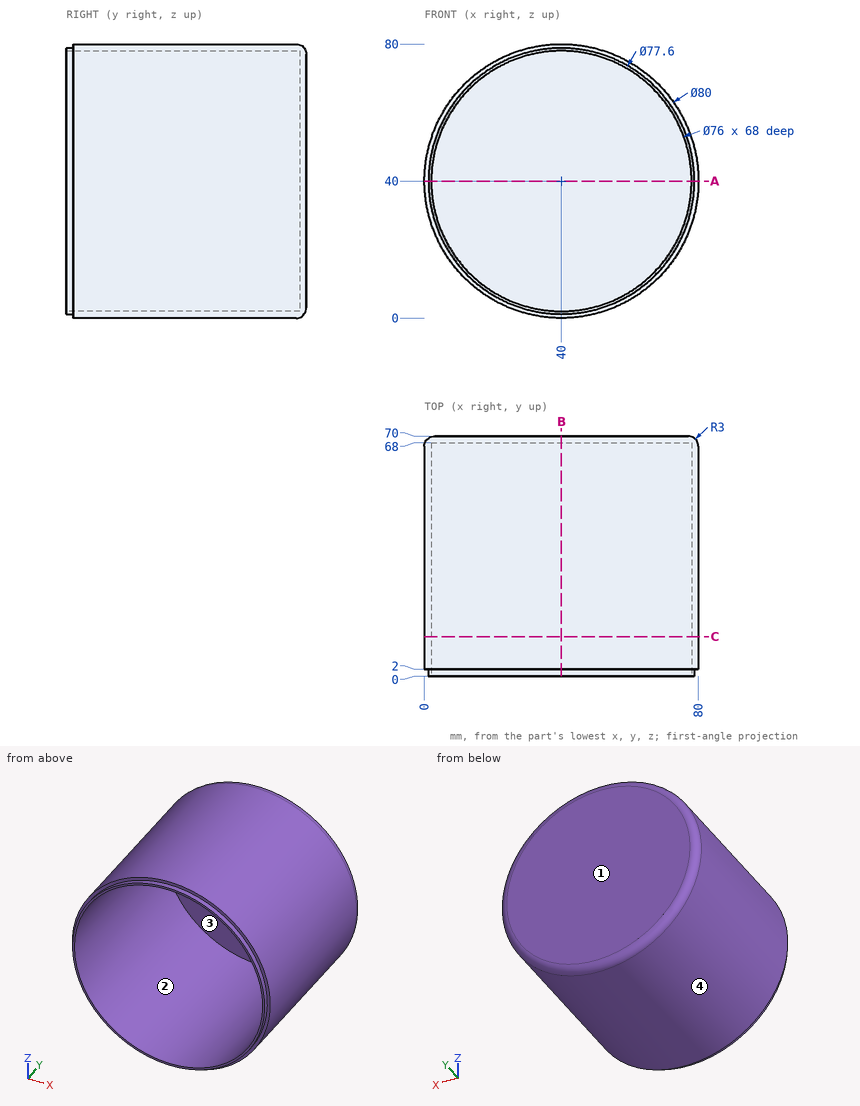
Design review of the part shown in the three views and the two pictorial views. Dimensions are in mm from the part's minimum x, y and z. Round coordinates to 2 decimals unless told otherwise and drop trailing zeros. Write each loop counter-clockwise with the first axis right and the second up, starting at its lowest first coordinate (ties: lowest second). Pieces come first, ordered by that corner, then holes.
Item 1: Consider section B-B on x = 40. Give the boundary of the cut face in (y, z), and give its area (3 significant figures).
Item 2: Wall thickness on L1, parallel to X at y = 27.5, z = 40; L2, parallel to Y at x = 33.5, z = 16; L3, parallel to X at y = 9, z = 32: over which ranges is each line inside the solid? List them lowest first.
Item 3: Consider section C-C on y = 11.5. Give the boundary of the cut face in (x, z).
Item 4: For pin 1 Ø10 at (x, y) = (30, 36) entering from +Z; pin 2 Ø12 at (x, z) = (63.5, 44.5) entering from -Y; pin 3 Ø12 at (y, z) = (46.5, 21) entering from -X, all flat-tipped, find the tip position at first contact; note any pin that passes through.
Item 5: Draft analysis for pull direction X (two halves, no side actions). For the marked faces 1, 2, 3 and 4, state which applies: released by +X, released by -X, zero draft, split by the parting line, or undercut.
Item 6: Consider section A-A on z = 40. Give the boundary of the cut face in (x, y).
Check values:
1. outline: (0, 1.2) - (2, 1.2) - (2, 0) - (67, 0) arc R3 ccw to (70, 3) - (70, 77) arc R3 ccw to (67, 80) - (2, 80) - (2, 78.8) - (0, 78.8) - (0, 78) - (68, 78) - (68, 2) - (0, 2) - close
1. area: 423 mm2
2. L1: x = 0 to 2, 78 to 80
2. L2: y = 68 to 70
2. L3: x = 0.81 to 2.85, 77.15 to 79.19
3. outline: circle Ø80 at (40, 40); hole circle Ø76 at (40, 40)
4. pin 1: stops at z = 79.69
4. pin 2: stops at y = 68
4. pin 3: stops at x = 2.17
5. face 1: zero draft
5. face 2: undercut
5. face 3: undercut
5. face 4: split by the parting line
6. outline: (0, 2) - (1.2, 2) - (1.2, 0) - (2, 0) - (2, 68) - (78, 68) - (78, 0) - (78.8, 0) - (78.8, 2) - (80, 2) - (80, 67) arc R3 ccw to (77, 70) - (3, 70) arc R3 ccw to (0, 67) - close
